Geometry check sheet. Reference: drawing and pictorial views, mm from the part's lowest x, y, z. Round coordinates to 2 decimals unless told otherwise and drop trailing zeros. Loops run counter-clockwise (first coordinate to the right, second up) from the corner with the lowest first, then second, coordinate; pieces in that order, holes last. Notation, with made-up numbers: (60.25, -24.5) - (94.25, -24.5) arc R21 ccw to (94.25, -16.5) - close; hole circle Ø7 at (21, 76.5). An arc over 180 degrees is marked (long way). Put each result on its own line as item: value. Start each with the question number.
Item 1: Gauge pin test, flat ends, axial feed: pin 1 Ø5 at (x, z) = (8, 16) entering from -Y; pin 2 Ø2 at (x, z) = (1.5, 60) entering from +Y; pin 3 Ø3.5 at (x, z) = (6, 95.5) entering from +Y. Record the tip position at first contact, or that the pin passes through.
Item 2: Material ranges on line 1 along Z through (x, y) = (3.25, 8); line 2 along Y through (x, z) = (8, 19.5); line 3 along X through (y, z) = (5.25, 76.5), recorded low to high.
Item 3: Section check A-A, the plane x = 5. Record the cut outline in (y, z).
Item 4: Section check B-B, the plane z = 88. Record the cut outline in (x, y), and give its area (3 significant figures).
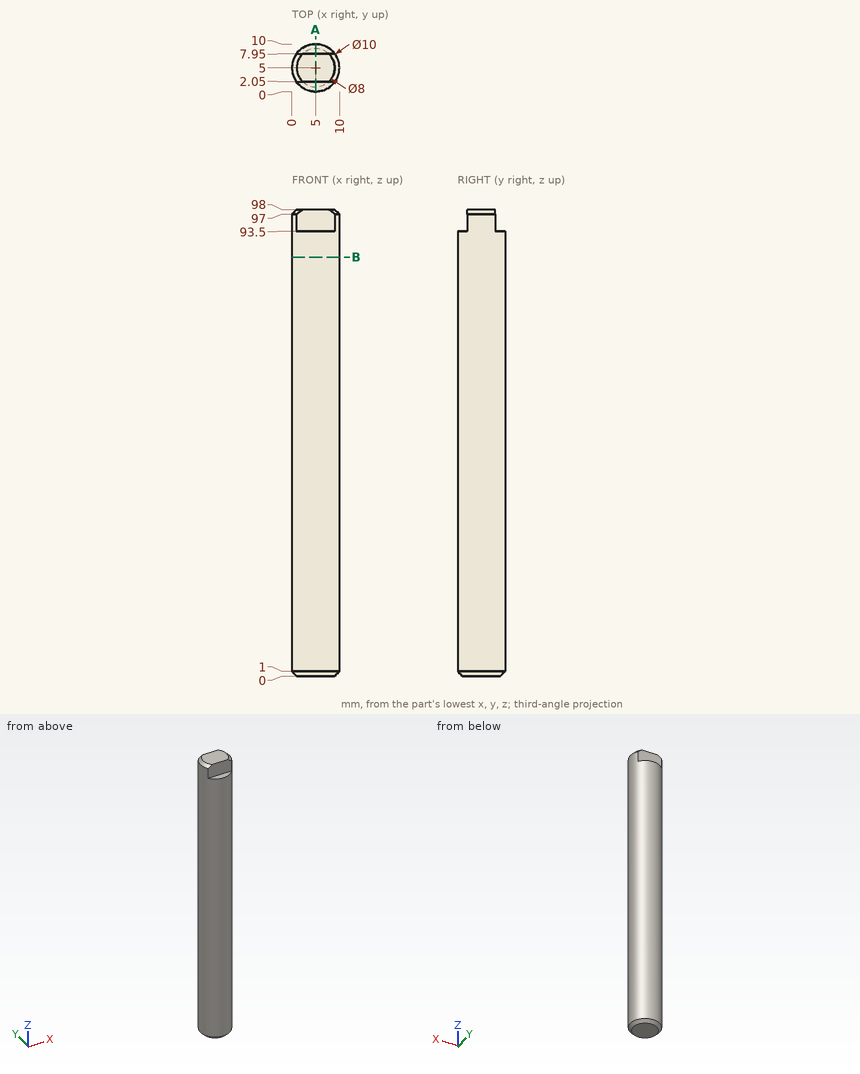
Check result:
1. pin 1: y = 0.03
1. pin 2: y = 9.33
1. pin 3: y = 7.95
2. line 1: 0 to 93.5
2. line 2: 1 to 9
2. line 3: 0.01 to 9.99
3. outline: (0, 1) - (1, 0) - (9, 0) - (10, 1) - (10, 93.5) - (7.95, 93.5) - (7.95, 98) - (2.05, 98) - (2.05, 93.5) - (0, 93.5) - close
4. outline: circle Ø10 at (5, 5)
4. area: 78.5 mm²
